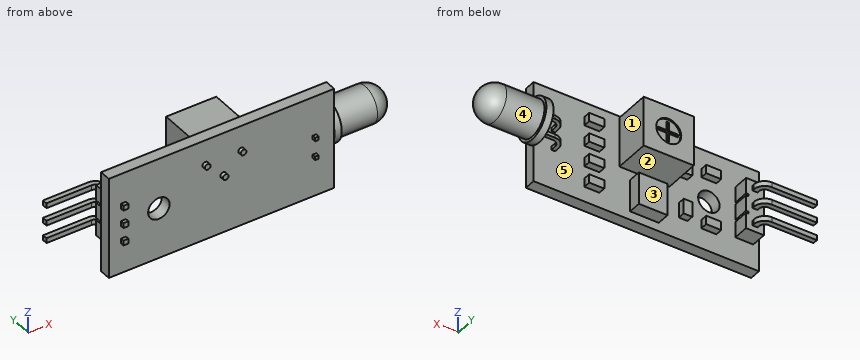
```python
from build123d import *

# Parameters (mm, degrees)
SKETCH_1_W             = 31.5
SKETCH_1_H             = 14.2
SKETCH_1_R             = 1.5
EXTRUDE_1_DEPTH        = 1.6
SKETCH_2_W             = 7
SKETCH_2_H             = 7
EXTRUDE_2_DEPTH        = 5
SKETCH_3_R             = 1.75
CUT_EXTRUDE_1_DEPTH    = 0.2
CUT_EXTRUDE_2_DEPTH    = 0.3
SKETCH_6_W             = 4
SKETCH_6_H             = 4.5
EXTRUDE_3_DEPTH        = 1.8
SKETCH_7_W             = 2.1
SKETCH_7_H             = 1.2
SKETCH_7_W_2           = 1.2
SKETCH_7_H_2           = 2.1
EXTRUDE_4_DEPTH        = 1
EXTRUDE_START          = 1.6
EXTRUDE_5_DEPTH        = 0.5
PATTERN_LINEAR_1_COUNT = 2
PATTERN_LINEAR_1_PITCH = 2.7
EXTRUDE_6_DEPTH        = 0.35
PATTERN_LINEAR_2_COUNT = 2
PATTERN_LINEAR_2_PITCH = 2.5
PATTERN_LINEAR_3_COUNT = 2
PATTERN_LINEAR_3_PITCH = 2.5
SKETCH_12_W            = 2.5
SKETCH_12_H            = 2.2
SKETCH_12_W_2          = 1.8
SKETCH_12_H_2          = 0.3
EXTRUDE_7_DEPTH        = 2.2
SKETCH_13_R            = 0.4
EXTRUDE_8_DEPTH        = 0.5


with BuildPart() as part:
    # Эскиз1 → Бобышка-Вытянуть1 (new body)
    with BuildSketch(Plane(origin=(0, 0, 0), x_dir=(1, 0, 0), z_dir=(0, 1, 0))):
        Rectangle(SKETCH_1_W, SKETCH_1_H)
        with Locations(Location((-8.75, 0, 0), (0, 0, 270))):
            Circle(SKETCH_1_R, mode=Mode.SUBTRACT)
    extrude(amount=EXTRUDE_1_DEPTH)

    # Эскиз2 → Бобышка-Вытянуть2 (add)
    with BuildSketch(Plane(origin=(0, 1.6, 0), x_dir=(1, 0, 0), z_dir=(0, 1, 0))):
        with Locations((0.25, -3.4)):
            Rectangle(SKETCH_2_W, SKETCH_2_H)
    extrude(amount=EXTRUDE_2_DEPTH)

    # Эскиз3 → Вырез-Вытянуть1 (cut)
    with BuildSketch(Plane(origin=(0, 6.6, 0), x_dir=(1, 0, 0), z_dir=(0, 1, 0))):
        with Locations(Location((0.25, -3.4, 0), (0, 0, 270))):
            Circle(SKETCH_3_R)
    extrude(amount=-CUT_EXTRUDE_1_DEPTH, mode=Mode.SUBTRACT)

    # Эскиз4 → Вырез-Вытянуть2 (cut)
    with BuildSketch(Plane(origin=(0, 6.4, 0), x_dir=(1, 0, 0), z_dir=(0, 1, 0))):
        Polygon((0.05, -2), (0.45, -2), (0.45, -3.2), (1.65, -3.2), (1.65, -3.6), (0.45, -3.6), (0.45, -4.8), (0.05, -4.8), (0.05, -3.6), (-1.15, -3.6), (-1.15, -3.2), (0.05, -3.2), align=None)
    extrude(amount=-CUT_EXTRUDE_2_DEPTH, mode=Mode.SUBTRACT)

    # Эскиз6 → Бобышка-Вытянуть3 (add)
    with BuildSketch(Plane(origin=(0, 1.6, 0), x_dir=(1, 0, 0), z_dir=(0, 1, 0))):
        with Locations((0.25, 3.65)):
            Rectangle(SKETCH_6_W, SKETCH_6_H)
    extrude(amount=EXTRUDE_3_DEPTH)

    # Эскиз7 → Бобышка-Вытянуть4 (add)
    with BuildSketch(Plane(origin=(0, 1.6, 0), x_dir=(1, 0, 0), z_dir=(0, 1, 0))):
        with Locations((7.6, 1.466666667)):
            Rectangle(SKETCH_7_W, SKETCH_7_H)
        with Locations((7.6, 4.4)):
            Rectangle(SKETCH_7_W, SKETCH_7_H)
        with Locations((-8.75, 3.65)):
            Rectangle(SKETCH_7_W, SKETCH_7_H)
        with Locations((-5.15, 2.95)):
            Rectangle(SKETCH_7_W_2, SKETCH_7_H_2)
        with Locations((-5.15, -2.95)):
            Rectangle(SKETCH_7_W_2, SKETCH_7_H_2)
        with Locations((-8.75, -3.65)):
            Rectangle(SKETCH_7_W, SKETCH_7_H)
        with Locations((7.6, -4.4)):
            Rectangle(SKETCH_7_W, SKETCH_7_H)
        with Locations((7.6, -1.466666667)):
            Rectangle(SKETCH_7_W, SKETCH_7_H)
    extrude(amount=EXTRUDE_4_DEPTH)

    # Эскиз9 → Бобышка-Вытянуть5 (add)
    with BuildSketch(Plane.XY.offset(EXTRUDE_START)):
        with BuildLine():
            Line((12.75, 2.3), (12.75, -0.5))
            Line((12.75, -0.5), (13.25, -0.5))
            Line((13.25, -0.5), (13.25, 2.3))
            ThreePointArc((13.25, 2.3), (13.542893219, 3.007106781), (14.25, 3.3))
            Line((14.25, 3.3), (16.25, 3.3))
            Line((16.25, 3.3), (16.25, 3.8))
            Line((16.25, 3.8), (14.25, 3.8))
            ThreePointArc((14.25, 3.8), (13.189339828, 3.360660172), (12.75, 2.3))
        make_face()
    extrude_5 = extrude(amount=-EXTRUDE_5_DEPTH)

    # Линейный массив1: Бобышка-Вытянуть5 ×2
    with Locations(*[(0, 0, -i * PATTERN_LINEAR_1_PITCH) for i in range(1, PATTERN_LINEAR_1_COUNT)]):
        add(extrude_5)

    # Эскиз10 → Повернуть1 (revolve)
    with BuildSketch(Plane.XY, mode=Mode.PRIVATE) as revolve_1_sk:
        with BuildLine():
            Line((16.25, 3.55), (16.25, 6.45))
            Line((16.25, 6.45), (17.25, 6.45))
            Line((17.25, 6.45), (17.25, 6.05))
            Line((17.25, 6.05), (22.53, 6.05))
            ThreePointArc((22.53, 6.05), (24.297766953, 5.317766953), (25.03, 3.55))
            Line((25.03, 3.55), (16.25, 3.55))
        make_face()
    revolve(revolve_1_sk.sketch.rotate(Axis((16.25, 3.55, 0), (1, 0, 0)), 90), axis=Axis((16.25, 3.55, 0), (1, 0, 0)))

    # Эскиз11 → Бобышка-Вытянуть6 (add, symmetric)
    with BuildSketch(Plane.XY):
        with BuildLine():
            Line((-13.35, -0.5), (-14.05, -0.5))
            Line((-14.05, -0.5), (-14.05, 4.1))
            ThreePointArc((-14.05, 4.1), (-14.284314575, 4.665685425), (-14.85, 4.9))
            Line((-14.85, 4.9), (-21.15, 4.9))
            Line((-21.15, 4.9), (-21.15, 5.6))
            Line((-21.15, 5.6), (-14.85, 5.6))
            ThreePointArc((-14.85, 5.6), (-13.789339828, 5.160660172), (-13.35, 4.1))
            Line((-13.35, 4.1), (-13.35, -0.5))
        make_face()
    extrude_6 = extrude(amount=EXTRUDE_6_DEPTH, both=True)

    # Линейный массив2: Бобышка-Вытянуть6 ×2
    with Locations(*[(0, 0, i * PATTERN_LINEAR_2_PITCH) for i in range(1, PATTERN_LINEAR_2_COUNT)]):
        add(extrude_6)

    # Линейный массив3: Бобышка-Вытянуть6 ×2
    with Locations(*[(0, 0, -i * PATTERN_LINEAR_3_PITCH) for i in range(1, PATTERN_LINEAR_3_COUNT)]):
        add(extrude_6)

    # Эскиз12 → Бобышка-Вытянуть7 (add)
    with BuildSketch(Plane(origin=(0, 1.6, 0), x_dir=(1, 0, 0), z_dir=(0, 1, 0))):
        with Locations((-13.7, 2.5)):
            Rectangle(SKETCH_12_W, SKETCH_12_H)
        with Locations((-13.7, 1.25)):
            Rectangle(SKETCH_12_W_2, SKETCH_12_H_2)
        with Locations((-13.7, 0)):
            Rectangle(SKETCH_12_W, SKETCH_12_H)
        with Locations((-13.7, -1.25)):
            Rectangle(SKETCH_12_W_2, SKETCH_12_H_2)
        with Locations((-13.7, -2.5)):
            Rectangle(SKETCH_12_W, SKETCH_12_H)
    extrude(amount=EXTRUDE_7_DEPTH)

    # Эскиз13 → Бобышка-Вытянуть8 (add)
    with BuildSketch(Plane.XZ):
        with Locations(Location((-2.25, 3.6, 0), (0, 0, 90))):
            Circle(SKETCH_13_R)
        with Locations(Location((0.25, 1.1, 0), (0, 0, 90))):
            Circle(SKETCH_13_R)
        with Locations(Location((2.75, 3.6, 0), (0, 0, 90))):
            Circle(SKETCH_13_R)
    extrude(amount=EXTRUDE_8_DEPTH)


solid = part.part
```
The listing builds one solid part. Answer for the finished solid, in the listing's coordinates (mm). Face numbers are marked on the shaded views. A direction names the side the tool comes from. Coordinates: 2 decimals unless noted, no trailing zeros. Order: outer loops, then holes, each group sorted by start corner. A loop starts at its lowest first (then second) coordinate and runs counter-clockwise, first axis right, second up. Notation, with made-up numbers: M -10.5,-30.5 L -2.5,-30.5 A14 ccw -2.5,-11.5 Z; hole C 52,46.25 d9. An arc over 180 degrees is marked long. Answer as a JSON object with one key per item and string values. Group by question number.
1. Section C-C on x = -2.25 is taken. Write down the section's boundary in (y, z).
2. Section B-B on x = -8.75 is taken. Write down the section's boundary in (y, z), then the cut area to 3 significant figures.
3. Section D-D on x = -17.5 is taken. Write down the section's boundary in (y, z), then the cut area to 3 significant figures.
4. Determine the mould class of the marked faces 4 and 5 for opening direction X: released by +X, released by -X, zero draft, split by the parting line, or undercut.
5. Section A-A on x = 15 is taken. Write down the section's boundary in (y, z), then the cut area to 3 significant figures.
6. A tool of negligible diameter and unlimited length cuts with its end or side. For the marked faces 1, 2 and 3, from which of +Z, -Z, +X, -X, +Y, -Y can it reach the whole face along a straight path? Write none if from no direction.
7. Straight lines are drawn through the part: line 1 (X direction, y = 1, z = 0); line 2 (X direction, y = 2.5, z = 3); line 3 (X direction, y = 0.45, z = 0). For each, find the intervals that lie inside material, in ascending order.
8. Flat-ended cylindrical pins translate along their axes: P1, Ø0.6, axis at y = 0, z = -2.5, coming from the +X side; P2, Ø2, axis at y = 1.5, z = 4.5, coming from the -X side; P3, Ø1.1, axis at y = 2.5, z = -4, coming from the -X side. Find the tip coordinate at first contact, or state that the pin passes through.
Values follow:
{
 "1": {"outline": "M -0.5,3.2 L 0,3.2 L 0,-7.1 L 1.6,-7.1 L 1.6,-0.1 L 6.6,-0.1 L 6.6,6.9 L 1.6,6.9 L 1.6,7.1 L 0,7.1 L 0,4 L -0.5,4 Z"},
 "2": {"outline": "M 0,-7.1 L 1.6,-7.1 L 1.6,-4.25 L 2.6,-4.25 L 2.6,-3.05 L 1.6,-3.05 L 1.6,-1.5 L 0,-1.5 Z; M 0,1.5 L 1.6,1.5 L 1.6,3.05 L 2.6,3.05 L 2.6,4.25 L 1.6,4.25 L 1.6,7.1 L 0,7.1 Z", "area": "20.3 mm2"},
 "3": {"outline": "M 4.9,-2.85 L 5.6,-2.85 L 5.6,-2.15 L 4.9,-2.15 Z; M 4.9,-0.35 L 5.6,-0.35 L 5.6,0.35 L 4.9,0.35 Z; M 4.9,2.15 L 5.6,2.15 L 5.6,2.85 L 4.9,2.85 Z", "area": "1.47 mm2"},
 "4": {"face 4": "zero draft", "face 5": "undercut"},
 "5": {"outline": "M 0,-7.1 L 1.6,-7.1 L 1.6,7.1 L 0,7.1 Z; M 3.3,-1.6 L 3.8,-1.6 L 3.8,-1.1 L 3.3,-1.1 Z; M 3.3,1.1 L 3.8,1.1 L 3.8,1.6 L 3.3,1.6 Z", "area": "23.2 mm2"},
 "6": {"face 1": "+Z, -Z, +Y", "face 2": "+Y", "face 3": "-Z, +Y"},
 "7": {"line 1": "-15.75 to -10.25, -7.25 to 15.75, 16.25 to 17.25", "line 2": "-14.95 to -12.45, -5.75 to -4.55, -3.25 to 3.75", "line 3": "-15.75 to -10.25, -7.25 to 15.75"},
 "8": {"P1": "x = 15.75", "P2": "x = -15.75", "P3": "x = -14.95"}
}
